```python
from build123d import *

# Parameters (mm, degrees)
SKETCH1_W                 = 68.58
SKETCH1_H                 = 68.58
BASE_EXTRUDE_DEPTH        = 81.026
SIDE_FILLETS_R            = 12.7
TOP_CUT_DEPTH             = 5.08
TOP_FACE_FILLET_R         = 1.27
SKETCH4_R                 = 6.35
TERMINALS_DEPTH           = 15.24
TERMINALS_DRAFT           = 5
TERMINALS_PROFILE_2_DEPTH = 15.24
TERMINALS_PROFILE_2_DRAFT = 5


with BuildPart() as part:
    # Sketch1 → Base Extrude (new body)
    with BuildSketch(Plane(origin=(0, 0, 0), x_dir=(1, 0, 0), z_dir=(0, 1, 0))):
        Rectangle(SKETCH1_W, SKETCH1_H)
    extrude(amount=BASE_EXTRUDE_DEPTH)

    # Side Fillets
    side_fillets_edges = [part.edges().sort_by_distance(p)[0] for p in [
        (34.29, 40.513, 34.29),
        (-34.29, 40.513, 34.29),
        (-34.29, 40.513, -34.29),
        (34.29, 40.513, -34.29),
    ]]
    fillet(side_fillets_edges, radius=SIDE_FILLETS_R)

    # Sketch3 → Top Cut (cut)
    with BuildSketch(Plane(origin=(0, 81.026, 0), x_dir=(1, 0, 0), z_dir=(0, 1, 0))):
        with BuildLine():
            Line((21.59, 30.48), (-21.59, 30.48))
            ThreePointArc((-21.59, 30.48), (-27.876179285, 27.876179285), (-30.48, 21.59))
            Line((-30.48, 21.59), (-30.48, -21.59))
            ThreePointArc((-30.48, -21.59), (-27.876179285, -27.876179285), (-21.59, -30.48))
            Line((-21.59, -30.48), (21.59, -30.48))
            ThreePointArc((21.59, -30.48), (27.876179285, -27.876179285), (30.48, -21.59))
            Line((30.48, -21.59), (30.48, 21.59))
            ThreePointArc((30.48, 21.59), (27.876179285, 27.876179285), (21.59, 30.48))
        make_face()
    extrude(amount=-TOP_CUT_DEPTH, mode=Mode.SUBTRACT)

    # Top Face Fillet
    top_face_fillet_edges = [part.edges().sort_by_distance(p)[0] for p in [
        (-34.29, 81.026, 0),
        (0, 81.026, -34.29),
        (34.29, 81.026, 0),
        (0, 81.026, 34.29),
        (-30.570256121, 81.026, 30.570256121),
        (30.570256121, 81.026, 30.570256121),
        (30.570256121, 81.026, -30.570256121),
        (-30.570256121, 81.026, -30.570256121),
        (27.876179285, 81.026, -27.876179285),
        (0, 81.026, -30.48),
        (-27.876179285, 81.026, -27.876179285),
        (-30.48, 81.026, 0),
        (-27.876179285, 81.026, 27.876179285),
        (0, 81.026, 30.48),
        (27.876179285, 81.026, 27.876179285),
        (30.48, 81.026, 0),
    ]]
    fillet(top_face_fillet_edges, radius=TOP_FACE_FILLET_R)


with BuildPart() as terminals_tool:
    # Sketch4 → Terminals (with draft: the straight prism first)
    with BuildSketch(Plane(origin=(0, 75.946, 0), x_dir=(1, 0, 0), z_dir=(0, 1, 0))):
        Circle(SKETCH4_R)
    extrude(amount=TERMINALS_DEPTH)
    # Terminals: the draft: its side faces are tilted about the plane it starts from
    terminals_sides = [terminals_tool.faces().sort_by_distance(p)[0] for p in [
        (-6.35, 83.566, 0),
    ]]
    draft(terminals_sides, Plane(origin=(0, 75.946, 0), x_dir=(1, 0, 0), z_dir=(0, 1, 0)), TERMINALS_DRAFT)


with BuildPart() as part_1:
    add(part.part)

    # Terminals: add terminals_tool
    add(terminals_tool.part)


with BuildPart() as terminals_profile_2_tool:
    # Sketch4 → Terminals profile 2 (with draft: the straight prism first)
    with BuildSketch(Plane(origin=(0, 75.946, 0), x_dir=(1, 0, 0), z_dir=(0, 1, 0))):
        with Locations((-17.960512242, 17.960512242)):
            Circle(SKETCH4_R)
    extrude(amount=TERMINALS_PROFILE_2_DEPTH)
    # Terminals profile 2: the draft: its side faces are tilted about the plane it starts from
    terminals_profile_2_sides = [terminals_profile_2_tool.faces().sort_by_distance(p)[0] for p in [
        (-24.310512242, 83.566, -17.960512242),
    ]]
    draft(terminals_profile_2_sides, Plane(origin=(0, 75.946, 0), x_dir=(1, 0, 0), z_dir=(0, 1, 0)), TERMINALS_PROFILE_2_DRAFT)


with BuildPart() as part_2:
    add(part_1.part)

    # Terminals profile 2: add terminals_profile_2_tool
    add(terminals_profile_2_tool.part)


solid = part_2.part
```
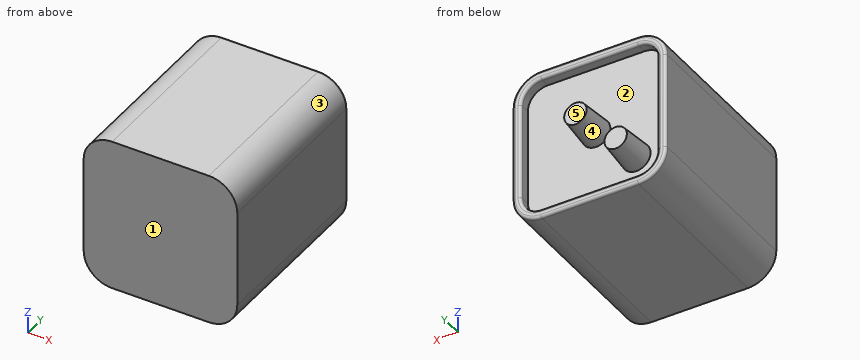
Work out the finished part from the listing and answer in its coordinate system (mm). Face numbers are marked on the shaded views. A direction names the side the tool comes from. Give positions to 0.01 mm unless a question says otherwise; leave off trailing zeros. Loops run counter-clockwise (first coordinate to the right, second up) from the corner with the lowest first, then second, coordinate; pieces in that order, holes last. Notation, with made-up numbers: M 65.5,57.25 L 95.5,57.25 A18 cw 95.5,71.25 Z; hole C 33,44.5 d6. An arc over 180 degrees is marked long. One line per item, written item: value. Start each with the question number.
1. Determine the mould class of the marked faces 3, 4 and 5 for opening direction X: released by +X, released by -X, zero draft, split by the parting line, or undercut.
2. Find the intervals of material crossed by probe 1 along Z at (x, y) = (-22, 76); probe 2 along Y at (x, z) = (0, 30); probe 3 along Z at (x, y) = (24, 79.5), in increasing order.
3. Find section A-A (x = 0). Give the vertices of the cut face in (y, z), and give its area (3 significant figures).
4. Which of the six approach directions +Z, -Z, +X, -X, +Y, -Y give full straight-line access (tool end or side, diameter ignored) to the marked faces 1 and 2?
5. Find section D-D (x = 18.5). Give the vertices of the cut face in (y, z), and give its area (3 significant figures).
6. Each of these flat-tipped pins is pushed along its axis until it touches: P1, Ø4, axis at x = 22.5, z = 13, coming from the +Y side; P2, Ø2, axis at x = 26, y = 42.5, coming from the -Z side. Where does it stop, or does it pass through?
7. Find section C-C (y = 18). Give the vertices of the cut face in (x, z).
8. Find section B-B (z = 0). Give the vertices of the cut face in (x, y), and give its area (3 significant figures).
Reported:
1. face 3: released by +X
1. face 4: undercut
1. face 5: zero draft
2. probe 1: z = -34.28 to -30.47, -22.85 to -13.07, 30.47 to 34.28
2. probe 2: y = 0 to 75.95
2. probe 3: z = -34.06 to -30.15, 30.15 to 34.06
3. outline: M 0,-34.29 L 79.76,-34.29 A1.27 ccw 81.03,-33.02 L 81.03,-31.75 A1.27 ccw 79.76,-30.48 L 75.95,-30.48 L 75.95,-6.35 L 91.19,-5.02 L 91.19,5.02 L 75.95,6.35 L 75.95,30.48 L 79.76,30.48 A1.27 ccw 81.03,31.75 L 81.03,33.02 A1.27 ccw 79.76,34.29 L 0,34.29 Z
3. area: 5,420 mm²
4. face 1: +Z, -Z, +X, -X, -Y
4. face 2: +Y
5. outline: M 0,-34.29 L 79.76,-34.29 A1.27 ccw 81.03,-33.02 L 81.03,-31.75 A1.27 ccw 79.76,-30.48 L 75.95,-30.48 L 75.95,30.48 L 79.76,30.48 A1.27 ccw 81.03,31.75 L 81.03,33.02 A1.27 ccw 79.76,34.29 L 0,34.29 Z
5. area: 5,250 mm²
6. P1: stops at y = 75.95
6. P2: stops at z = -33.82
7. outline: M -34.29,-21.59 A12.7 ccw -21.59,-34.29 L 21.59,-34.29 A12.7 ccw 34.29,-21.59 L 34.29,21.59 A12.7 ccw 21.59,34.29 L -21.59,34.29 A12.7 ccw -34.29,21.59 Z
8. outline: M -34.29,0 L 34.29,0 L 34.29,79.76 A1.27 ccw 33.02,81.03 L 31.75,81.03 A1.27 ccw 30.48,79.76 L 30.48,75.95 L 6.35,75.95 L 5.02,91.19 L -5.02,91.19 L -6.35,75.95 L -30.48,75.95 L -30.48,79.76 A1.27 ccw -31.75,81.03 L -33.02,81.03 A1.27 ccw -34.29,79.76 Z
8. area: 5,420 mm²
